Part model, mm, in its own coordinate system. Face numbers are marked on the shaded views. A direction names the side the tool comes from. Round coordinates to 2 decimals unless told otherwise and drop trailing zeros. Loops run counter-clockwise (first coordinate to the right, second up) from the corner with the lowest first, then second, coordinate; pieces in that order, holes last. Notation, with made-up numbers: (74, 26.5) - (95, 26.5) arc R28 ccw to (95, 65.5) - close; hole circle Ø9 at (75, 55.5). An arc over 180 degrees is marked (long way). Put each result on its own line as item: value.
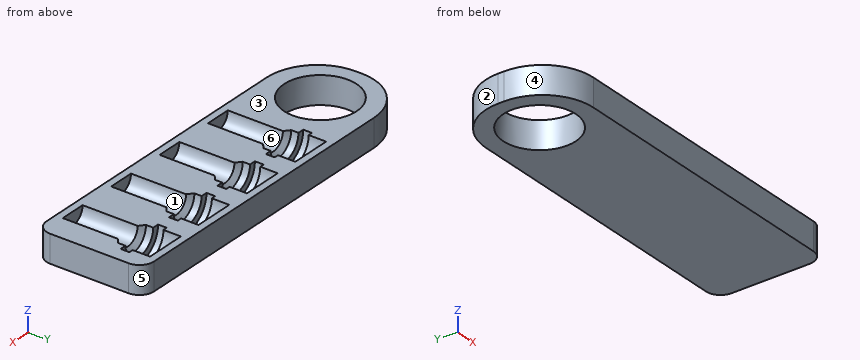
from build123d import *

# Parameters (mm, degrees)
F0_R     = 12.5
F1_DEPTH = 9.5


with BuildPart() as f1:
    # F0 (on Top) → F1 (new body)
    with BuildSketch(Plane.XY):
        with BuildLine():
            ThreePointArc((0, 17.5), (5.125631, 5.125631), (17.5, 0))
            Line((17.5, 0), (117.5, 0))
            ThreePointArc((117.5, 0), (121.035534, 1.464466), (122.5, 5))
            Line((122.5, 5), (122.5, 32))
            ThreePointArc((122.5, 32), (121.035534, 35.535534), (117.5, 37))
            Line((117.5, 37), (17.5, 37))
            ThreePointArc((17.5, 37), (5.125631, 31.874369), (0, 19.5))
            Line((0, 19.5), (0, 17.5))
        make_face()
        with Locations((17.5, 18.5)):
            Circle(F0_R, mode=Mode.SUBTRACT)
    extrude(amount=F1_DEPTH)

    # F2 (on face) → F3 (revolve, cut)
    with BuildSketch(Plane.XY.offset(9.5)):
        Polygon((109, 21.5), (109, 2.5), (113.5, 2.5), (113.5, 21.5), (115.3, 23), (115.3, 25.5), (117.5, 25.5), (117.5, 28.5), (116, 28.5), (116, 34.5), (109, 34.5), (109, 28.5), (109, 25.5), (109, 23), align=None)
    revolve(axis=Axis((109, 12, 9.5), (0, 1, 0)), mode=Mode.SUBTRACT)

    # F2 (on face) → F4 (revolve, cut)
    with BuildSketch(Plane.XY.offset(9.5)):
        Polygon((87, 21.5), (87, 2.5), (91.5, 2.5), (91.5, 21.5), (93.3, 23), (93.3, 25.5), (95.5, 25.5), (95.5, 28.5), (94, 28.5), (94, 34.5), (87, 34.5), (87, 28.5), (87, 25.5), (87, 23), align=None)
    revolve(axis=Axis((87, 12, 9.5), (0, 1, 0)), mode=Mode.SUBTRACT)

    # F2 (on face) → F5 (revolve, cut)
    with BuildSketch(Plane.XY.offset(9.5)):
        Polygon((65, 21.5), (65, 2.5), (69.5, 2.5), (69.5, 21.5), (71.3, 23), (71.3, 25.5), (73.5, 25.5), (73.5, 28.5), (72, 28.5), (72, 34.5), (65, 34.5), (65, 28.5), (65, 25.5), (65, 23), align=None)
    revolve(axis=Axis((65, 12, 9.5), (0, 1, 0)), mode=Mode.SUBTRACT)

    # F2 (on face) → F6 (revolve, cut)
    with BuildSketch(Plane.XY.offset(9.5)):
        Polygon((43, 21.5), (43, 2.5), (47.5, 2.5), (47.5, 21.5), (49.3, 23), (49.3, 25.5), (51.5, 25.5), (51.5, 28.5), (50, 28.5), (50, 34.5), (43, 34.5), (43, 28.5), (43, 25.5), (43, 23), align=None)
    revolve(axis=Axis((43, 12, 9.5), (0, 1, 0)), mode=Mode.SUBTRACT)


solid = f1.part
1. Band-saw the part on A-A (x = 87). List the corners of the cut face in (y, z), plus the area to 3 significant figures.
A:
outline: (0, 0) - (37, 0) - (37, 9.5) - (34.5, 9.5) - (34.5, 2.5) - (28.5, 2.5) - (28.5, 1) - (25.5, 1) - (25.5, 3.2) - (23, 3.2) - (21.5, 5) - (2.5, 5) - (2.5, 9.5) - (0, 9.5) - close
area: 175 mm²
2. Pin check, flat tips, straight feed: P1, Ø2, axis at y = 20.5, z = 2, coming from the -X side; P2, Ø4, axis at y = 27.5, z = 8.5, coming from the -X side. Stop position of each tip, or through.
A:
P1: stops at x = 0
P2: stops at x = 1.06
3. Two-plate mould, pull along Y, no slides. Class the marked faces 3, 4, 5 and 6: pulls with the +Y half, pulls with the -Y half, needs draft (parallel to the pull), parting line crosses it, or undercut.
A:
face 3: needs draft
face 4: pulls with the -Y half
face 5: pulls with the +Y half
face 6: undercut
4. Tool access for the marked faces 1 and 2: list every direction of +Z, -Z, +X, -X, +Y, -Y with a clear straight run to the whole face (end or side of a thin tool).
A:
face 1: +Z
face 2: +Z, -Z, -X, +Y
5. Band-saw the part on B-B (z = 7.5). Give the number of separate pieces and of enclosed holes in the cut face, plus the area to 3 significant figures.
A:
separate pieces: 1
enclosed holes: 5
area: 2,590 mm²
6. Probe line 1 along Y through (x, z) = (17.5, 5.25); line 2 along Y through (x, z) = (94, 6.75); line 3 along X through (y, z) = (29.5, 3.5). List the from-to ranges inside material, lowest first. Write a range as [from, to].
A:
line 1: y = [0, 6], [31, 37]
line 2: y = [0, 25.5], [28.5, 37]
line 3: x = [3.14, 11.56], [23.44, 39.39], [46.61, 61.39], [68.61, 83.39], [90.61, 105.39], [112.61, 122.5]
